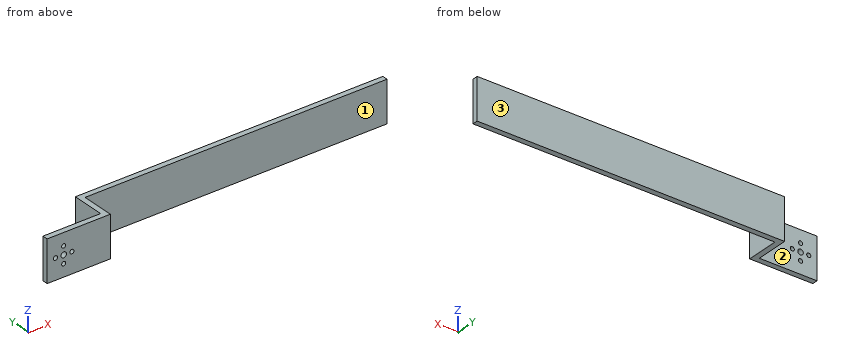
```python
from build123d import *

# Parameters (mm, degrees)
SKETCH1_W           = 46
SKETCH1_H           = 30
SKETCH1_R           = 1.5
SKETCH1_R_2         = 2
BOSS_EXTRUDE1_DEPTH = 4
SKETCH2_W           = 4
SKETCH2_H           = 30
BOSS_EXTRUDE2_DEPTH = 24
SKETCH3_W           = 30
SKETCH3_H           = 4
BOSS_EXTRUDE3_DEPTH = 220


with BuildPart() as part:
    # Sketch1 → Boss-Extrude1 (new body)
    with BuildSketch(Plane(origin=(0, 0, 0), x_dir=(1, 0, 0), z_dir=(0, 1, 0))):
        Rectangle(SKETCH1_W, SKETCH1_H)
        with Locations(Location((-17, 0, 0), (0, 0, 270))):
            Circle(SKETCH1_R, mode=Mode.SUBTRACT)
        with Locations(Location((-11, 6, 0), (0, 0, 270))):
            Circle(SKETCH1_R, mode=Mode.SUBTRACT)
        with Locations(Location((-5, 0, 0), (0, 0, 270))):
            Circle(SKETCH1_R, mode=Mode.SUBTRACT)
        with Locations(Location((-11, -6, 0), (0, 0, 270))):
            Circle(SKETCH1_R, mode=Mode.SUBTRACT)
        with Locations(Location((-11, 0, 0), (0, 0, 270))):
            Circle(SKETCH1_R_2, mode=Mode.SUBTRACT)
    extrude(amount=BOSS_EXTRUDE1_DEPTH)

    # Sketch2 → Boss-Extrude2 (add)
    with BuildSketch(Plane(origin=(0, 4, 0), x_dir=(1, 0, 0), z_dir=(0, 1, 0))):
        with Locations((21, 0)):
            Rectangle(SKETCH2_W, SKETCH2_H)
    extrude(amount=BOSS_EXTRUDE2_DEPTH)

    # Sketch3 → Boss-Extrude3 (add)
    with BuildSketch(Plane(origin=(23, 0, 0), x_dir=(0, 0, -1), z_dir=(1, 0, 0))):
        with Locations((0, 26)):
            Rectangle(SKETCH3_W, SKETCH3_H)
    extrude(amount=BOSS_EXTRUDE3_DEPTH)


solid = part.part
```
Check sheet for the modelled part. Datum: model origin and axes. Units: mm. Face numbers are marked on the shaded views. A direction names the side the tool comes from. Coordinates: 2 decimals unless noted, no trailing zeros. Write each loop counter-clockwise with the first axis right and the second up, starting at its lowest first coordinate (ties: lowest second). Pieces come first, ordered by that corner, then holes. Notation, with made-up numbers: (42.5, -31.5) -> (93.5, -31.5) arc R15 cw to (93.5, -23.5) -> close; hole circle Ø11 at (72, -3.5). An arc over 180 degrees is marked (long way). Use a Markdown table: item, result.
1. Go/stop test with flat-tipped pins: pin 1 Ø4 at (x, z) = (127, -1) entering from -Y; pin 2 Ø9 at (x, z) = (-8, 3) entering from +Y; pin 3 Ø2.5 at (x, z) = (-11, 6) entering from -Y; pin 4 Ø3 at (y, z) = (18, 2) entering from -X. Record where each tip stops, or that it passes through.
Reported:
| item | result |
|---|---|
| pin 1 | stops at y = 24 |
| pin 2 | stops at y = 4 |
| pin 3 | passes through |
| pin 4 | stops at x = 19 |
2. Scan lines: line 1 along X through (y, z) = (2.5, -6); line 2 along X through (y, z) = (1.2, 0); line 3 along X through (y, z) = (14.5, -7.25). Record each from-to range of solid material in increasing order.
Reported:
| item | result |
|---|---|
| line 1 | x = -23 to -12.5, -9.5 to 23 |
| line 2 | x = -23 to -18.5, -15.5 to -13, -9 to -6.5, -3.5 to 23 |
| line 3 | x = 19 to 23 |
3. Tool access check on the marked faces 1, 2 and 3. Record the directions out of +Z, -Z, +X, -X, +Y, -Y that give a thin tool (end or side, any length) a straight path to the whole face; none if there is none.
Reported:
| item | result |
|---|---|
| face 1 | +Z, -Z, +X, -Y |
| face 2 | +Z, -Z, -X, +Y |
| face 3 | +Z, -Z, +X, -X, +Y |
4. Sectioned sample at C-C (y = 16.25). Enter the section's corners in (x, z), plus the area to 3 significant figures.
Reported:
| item | result |
|---|---|
| outline | (19, -15) -> (23, -15) -> (23, 15) -> (19, 15) -> close |
| area | 120 mm2 |
5. Sectioned sample at B-B (x = 3.5). Enter the section's corners in (y, z).
Reported:
| item | result |
|---|---|
| outline | (0, -15) -> (4, -15) -> (4, 15) -> (0, 15) -> close |
6. Sectioned sample at A-A (z = 11). Enter the section's corners in (x, y).
Reported:
| item | result |
|---|---|
| outline | (-23, 0) -> (23, 0) -> (23, 24) -> (243, 24) -> (243, 28) -> (19, 28) -> (19, 4) -> (-23, 4) -> close |
